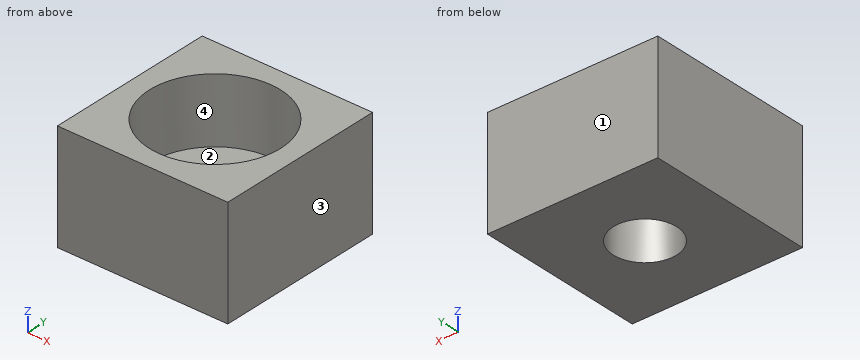
```python
from build123d import *

# Parameters (mm, degrees)
SKETCH_1_W          = 7.8
SKETCH_1_H          = 7.8
SKETCH_1_R          = 1.45
EXTRUDE_1_DEPTH     = 5
SKETCH_2_R          = 3
CUT_EXTRUDE_1_DEPTH = 3


with BuildPart() as part:
    # Эскиз1 → Бобышка-Вытянуть1 (new body)
    with BuildSketch(Plane.XY):
        Rectangle(SKETCH_1_W, SKETCH_1_H)
        Circle(SKETCH_1_R, mode=Mode.SUBTRACT)
    extrude(amount=EXTRUDE_1_DEPTH)

    # Эскиз2 → Вырез-Вытянуть1 (cut)
    with BuildSketch(Plane.XY.offset(5)):
        Circle(SKETCH_2_R)
    extrude(amount=-CUT_EXTRUDE_1_DEPTH, mode=Mode.SUBTRACT)


solid = part.part
```
Part model, mm, in its own coordinate system. Face numbers are marked on the shaded views. Round coordinates to 2 decimals unless told otherwise and drop trailing zeros. Loops run counter-clockwise (first coordinate to the right, second up) from the corner with the lowest first, then second, coordinate; pieces in that order, holes last.
Item 1: Drill centre lines: line 1 (Y direction, x = 0, z = 0.95); line 2 (Y direction, x = 0, z = 2.75). Where is each one in solid material? Low to high.
Item 2: Cut at D-D, the plane x = 2. Give the cut face in (y, z), then the cut area to 3 significant figures.
Item 3: Mould opens along Y. For the marked faces 1, 2, 3 and 4 say: +Y half, -Y half, draft (parallel to the pull), parting line (faces both ways), or undercut.
Item 4: Cut at C-C, the plane z = 4.2. Give the cut face in (x, y).
Item 5: Drop flat-ended pins along their axis: P1, Ø4, axis at x = 0, y = 0, coming from the +Z side; P2, Ø4, axis at x = -2.5, y = 0.5, coming from the +Z side; P3, Ø1.8, axis at x = -0.5, y = 0, coming from the +Z side. Give the stop position or say it passes through.
Item 6: Cut at A-A, the plane x = 0. Give the cut face in (y, z).
A:
1. line 1: y = -3.9 to -1.45, 1.45 to 3.9
1. line 2: y = -3.9 to -3, 3 to 3.9
2. outline: (-3.9, 0) - (3.9, 0) - (3.9, 5) - (2.24, 5) - (2.24, 2) - (-2.24, 2) - (-2.24, 5) - (-3.9, 5) - close
2. area: 25.6 mm2
3. face 1: +Y half
3. face 2: undercut
3. face 3: draft
3. face 4: undercut
4. outline: (-3.9, -3.9) - (3.9, -3.9) - (3.9, 3.9) - (-3.9, 3.9) - close; hole circle Ø6 at (0, 0)
5. P1: stops at z = 2
5. P2: stops at z = 5
5. P3: passes through
6. outline: (-3.9, 0) - (-1.45, 0) - (-1.45, 2) - (-3, 2) - (-3, 5) - (-3.9, 5) - close; (1.45, 0) - (3.9, 0) - (3.9, 5) - (3, 5) - (3, 2) - (1.45, 2) - close
